For this review, take the finished solid that the model builds, in its own axes (mm). Face numbers are marked on the shaded views. A direction names the side the tool comes from. Coordinates: 2 decimals unless noted, no trailing zeros. Write each loop counter-clockwise with the first axis right and the second up, starting at its lowest first coordinate (ties: lowest second). Pieces come first, ordered by that corner, then holes.
1) We need section C-C on x = 4. Write out the cut boundary in (y, z), then the cut area to 3 significant figures.
2) We need section A-A on z = -35. Write out the cut boundary in (x, y), then the cut area to 3 significant figures.
3) To check wall thickness, follow line 1 along X through (y, z) = (2.05, -35); line 2 along X through (y, z) = (8.25, -35); line 3 along X through (y, z) = (8.75, -14). State the ranges of each line that lie inside material, in increasing order.
4) Insertion check: P1, Ø10.5, axis at x = 0.5, z = -34, coming from the +Y side; P2, Ø4, axis at x = 23.5, y = 7, coming from the -Z side; P3, Ø7.5, axis at x = 0, z = -35, coming from the +Y side; P4, Ø5, axis at y = 5, z = -30.5, coming from the -X side. Each pin has a flat end and moves straight along its axis. Give the tip position at first contact, or say it passes through.
5) For the marked faces 5, 6 and 7, list the 3-axis set-ups (+Z, -Z, +X, -X, +Y, -Y) from which the entire face can be reached by the end or side of a thin tool; tool diameter is ignored.
6) We need section D-D on y = 1. Write out the cut boundary in (x, z).
7) We need section B-B on y = 8. Write out the cut boundary in (x, z), then the cut area to 3 significant figures.
8) Mouldability with a two-part tool opening along X and no side actions: class the marked faces 1, 2, 3 and 4 as pulls with the +X half, pulls with the -X half, needs draft (parallel to the pull), parting line crosses it, or undercut.
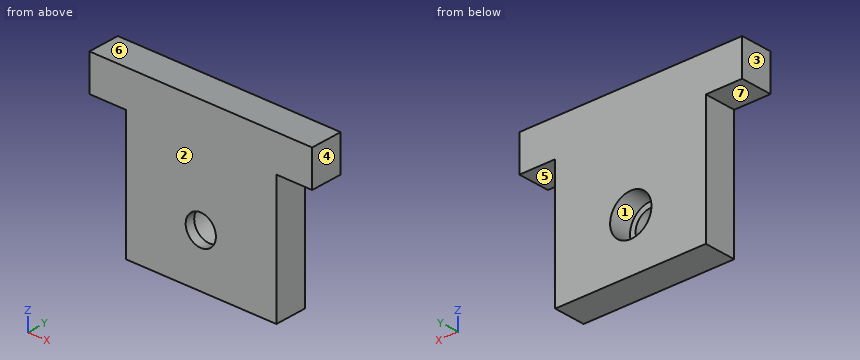
from build123d import *

# Parameters (mm, degrees)
BOSS_EXTRUDE1_DEPTH = 10
SKETCH2_R           = 6.5
CUT_EXTRUDE2_DEPTH  = 7
SKETCH5_R           = 4.75
CUT_EXTRUDE3_DEPTH  = 63.601101901


with BuildPart() as part:
    # Sketch1 → Boss-Extrude1 (new body)
    with BuildSketch(Plane(origin=(0, 0, 0), x_dir=(1, 0, 0), z_dir=(0, 1, 0))):
        Polygon((-23.571428571, 51.428571429), (23.752103043, 51.377146806), (23.752103043, 11.377146806), (35, 11.377146806), (35, 0), (-35, 0), (-35, 11.428571429), (-23.571428571, 11.428571429), align=None)
    extrude(amount=BOSS_EXTRUDE1_DEPTH)

    # Sketch2 → Cut-Extrude2 (cut)
    with BuildSketch(Plane(origin=(0, 10, 0), x_dir=(1, 0, 0), z_dir=(0, 1, 0))):
        with Locations(Location((0, 35, 0), (0, 0, 270))):
            Circle(SKETCH2_R)
    extrude(amount=-CUT_EXTRUDE2_DEPTH, mode=Mode.SUBTRACT)

    # Sketch5 → Cut-Extrude3 (cut, through all)
    with BuildSketch(Plane(origin=(0, 3, 0), x_dir=(1, 0, 0), z_dir=(0, 1, 0))):
        with Locations(Location((0, 35, 0), (0, 0, 270))):
            Circle(SKETCH5_R)
    extrude(amount=-CUT_EXTRUDE3_DEPTH, mode=Mode.SUBTRACT)


solid = part.part
Result:
1. outline: (0, -51.4) - (10, -51.4) - (10, -40.12) - (3, -40.12) - (3, -37.56) - (0, -37.56) - close; (0, -32.44) - (3, -32.44) - (3, -29.88) - (10, -29.88) - (10, 0) - (0, 0) - close
1. area: 427 mm2
2. outline: (-23.57, 0) - (-4.75, 0) - (-4.75, 3) - (-6.5, 3) - (-6.5, 10) - (-23.57, 10) - close; (4.75, 0) - (23.75, 0) - (23.75, 10) - (6.5, 10) - (6.5, 3) - (4.75, 3) - close
2. area: 354 mm2
3. line 1: x = -23.57 to -4.75, 4.75 to 23.75
3. line 2: x = -23.57 to -6.5, 6.5 to 23.75
3. line 3: x = -23.57 to 23.75
4. P1: stops at y = 3
4. P2: stops at z = -51.38
4. P3: passes through
4. P4: stops at x = -23.57
5. face 5: -Z, +X, +Y, -Y
5. face 6: +Z, +X, -X, +Y, -Y
5. face 7: -Z, -X, +Y, -Y
6. outline: (-35, -11.43) - (-23.57, -11.43) - (-23.57, -51.43) - (23.75, -51.38) - (23.75, -11.38) - (35, -11.38) - (35, 0) - (-35, 0) - close; hole circle Ø9.5 at (0, -35)
7. outline: (-35, -11.43) - (-23.57, -11.43) - (-23.57, -51.43) - (23.75, -51.38) - (23.75, -11.38) - (35, -11.38) - (35, 0) - (-35, 0) - close; hole circle Ø13 at (0, -35)
7. area: 2,560 mm2
8. face 1: undercut
8. face 2: needs draft
8. face 3: pulls with the -X half
8. face 4: pulls with the +X half
